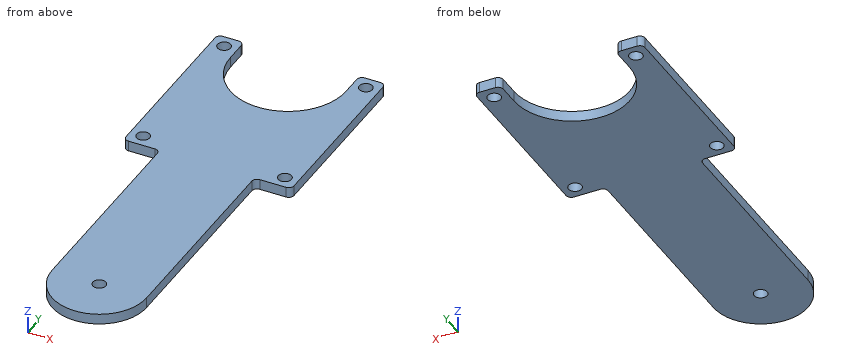
from build123d import *

# Parameters (mm, degrees)
SKETCH_1_R      = 1.25
EXTRUDE_1_DEPTH = 2


with BuildPart() as part:
    # 草圖1 → 填料-伸長1 (new body)
    with BuildSketch(Plane.XY):
        with BuildLine():
            Line((18.048613933, -20.404186252), (23.048613933, -20.404186252))
            ThreePointArc((23.048613933, -20.404186252), (23.755720714, -20.111293033), (24.048613933, -19.404186252))
            Line((24.048613933, -19.404186252), (24.048613933, -15.404186252))
            Line((24.048613933, -15.404186252), (24.048613933, -2.404186252))
            Line((24.048613933, -2.404186252), (24.048613933, 13.595813748))
            ThreePointArc((24.048613933, 13.595813748), (23.755720714, 14.302920529), (23.048613933, 14.595813748))
            Line((23.048613933, 14.595813748), (20.048613933, 14.595813748))
            ThreePointArc((20.048613933, 14.595813748), (19.341507152, 14.302920529), (19.048613933, 13.595813748))
            Line((19.048613933, 13.595813748), (19.048613933, 9.595813748))
            ThreePointArc((19.048613933, 9.595813748), (8.048613933, -1.404186252), (-2.951386067, 9.595813748))
            Line((-2.951386067, 9.595813748), (-2.951386067, 13.595813748))
            ThreePointArc((-2.951386067, 13.595813748), (-3.244279286, 14.302920529), (-3.951386067, 14.595813748))
            Line((-3.951386067, 14.595813748), (-6.951386067, 14.595813748))
            ThreePointArc((-6.951386067, 14.595813748), (-7.658492848, 14.302920529), (-7.951386067, 13.595813748))
            Line((-7.951386067, 13.595813748), (-7.951386067, -2.404186252))
            Line((-7.951386067, -2.404186252), (-7.951386067, -15.404186252))
            Line((-7.951386067, -15.404186252), (-7.951386067, -19.404186252))
            ThreePointArc((-7.951386067, -19.404186252), (-7.658492848, -20.111293033), (-6.951386067, -20.404186252))
            Line((-6.951386067, -20.404186252), (-1.951386067, -20.404186252))
            ThreePointArc((-1.951386067, -20.404186252), (-1.244279286, -20.697079471), (-0.951386067, -21.404186252))
            Line((-0.951386067, -21.404186252), (-0.951386067, -60.404186252))
            ThreePointArc((-0.951386067, -60.404186252), (8.048613933, -69.404186252), (17.048613933, -60.404186252))
            Line((17.048613933, -60.404186252), (17.048613933, -21.404186252))
            ThreePointArc((17.048613933, -21.404186252), (17.341507152, -20.697079471), (18.048613933, -20.404186252))
        make_face()
        with Locations((8.048613933, -60.404186252)):
            Circle(SKETCH_1_R, mode=Mode.SUBTRACT)
        with Locations((-5.451386067, -17.904186252)):
            Circle(SKETCH_1_R, mode=Mode.SUBTRACT)
        with Locations((-5.451386067, 12.095813748)):
            Circle(SKETCH_1_R, mode=Mode.SUBTRACT)
        with Locations((21.548613933, -17.904186252)):
            Circle(SKETCH_1_R, mode=Mode.SUBTRACT)
        with Locations((21.548613933, 12.095813748)):
            Circle(SKETCH_1_R, mode=Mode.SUBTRACT)
    extrude(amount=EXTRUDE_1_DEPTH)


solid = part.part
Work out the finished part from the listing and answer in its coordinate system (mm). Round coordinates to 2 decimals unless told otherwise and drop trailing zeros. Write each loop counter-clockwise with the first axis right and the second up, starting at its lowest first coordinate (ties: lowest second). Pieces come first, ordered by that corner, then holes. Notation, with made-up numbers: (30.25, -30.75) -> (74.25, -30.75) arc R20 cw to (74.25, -6.75) -> close; hole circle Ø11 at (66.5, -21). An arc over 180 degrees is marked (long way). Answer as CSV lines item,"result". Start each with the question number.
(1) The part is cut by section B-B, the plane x = 8. Give the vertices of the cut face in (y, z).
(2) The part is cut by section A-A, the plane z = 1.5. Give the vertices of the cut face in (x, y), then the cut area to 3 significant figures.
(3) Find the intervals of material crossed by probe 1 along Y at (x, z) = (-5.5, 0.45); probe 2 along Y at (x, z) = (21, 0.7); probe 3 along X at (y, z) = (-53.5, 1.8), in increasing order.
(4) Each of these flat-tipped pins is pushed along its axis until it touches: pin 1 (1 mm diameter, centred on x = 21, z = 1, fed in from -Y); pin 2 (0.6 mm diameter, centred on y = -46.5, z = 1, fed in from -X). Where does it stop, or does it pass through?
(5) The part is cut by section C-C, the plane y = -48. Give the vertices of the cut face in (x, z), then the cut area to 3 significant figures.
Output values:
1,outline,"(-69.4, 0) -> (-61.65, 0) -> (-61.65, 2) -> (-69.4, 2) -> close; (-59.16, 0) -> (-1.4, 0) -> (-1.4, 2) -> (-59.16, 2) -> close"
2,outline,"(-7.95, -19.4) arc R1 ccw to (-6.95, -20.4) -> (-1.95, -20.4) arc R1 cw to (-0.95, -21.4) -> (-0.95, -60.4) arc R9 ccw to (17.05, -60.4) -> (17.05, -21.4) arc R1 cw to (18.05, -20.4) -> (23.05, -20.4) arc R1 ccw to (24.05, -19.4) -> (24.05, 13.6) arc R1 ccw to (23.05, 14.6) -> (20.05, 14.6) arc R1 ccw to (19.05, 13.6) -> (19.05, 9.6) arc R11 cw to (-2.95, 9.6) -> (-2.95, 13.6) arc R1 ccw to (-3.95, 14.6) -> (-6.95, 14.6) arc R1 ccw to (-7.95, 13.6) -> close; hole circle Ø2.5 at (-5.45, -17.9); hole circle Ø2.5 at (-5.45, 12.1); hole circle Ø2.5 at (8.05, -60.4); hole circle Ø2.5 at (21.55, -17.9); hole circle Ø2.5 at (21.55, 12.1)"
2,area,"1,640 mm²"
3,probe 1,"y = -20.4 to -19.15, -16.66 to 10.85, 13.34 to 14.6"
3,probe 2,"y = -20.4 to -19.03, -16.78 to 10.97, 13.22 to 14.6"
3,probe 3,"x = -0.95 to 17.05"
4,pin 1,"stops at y = -20.4"
4,pin 2,"stops at x = -0.95"
5,outline,"(-0.95, 0) -> (17.05, 0) -> (17.05, 2) -> (-0.95, 2) -> close"
5,area,"36.0 mm²"
